Study the drawing (mm; zero at the part's minimum x, y, z) and answer. Round coordinates to 2 decimals unless told otherwise and drop trailing zeros. Write each loop counter-clockwise with the first axis right and the second up, starting at its lowest first coordinate (ties: lowest second). Pieces come first, ordered by that corner, then holes.
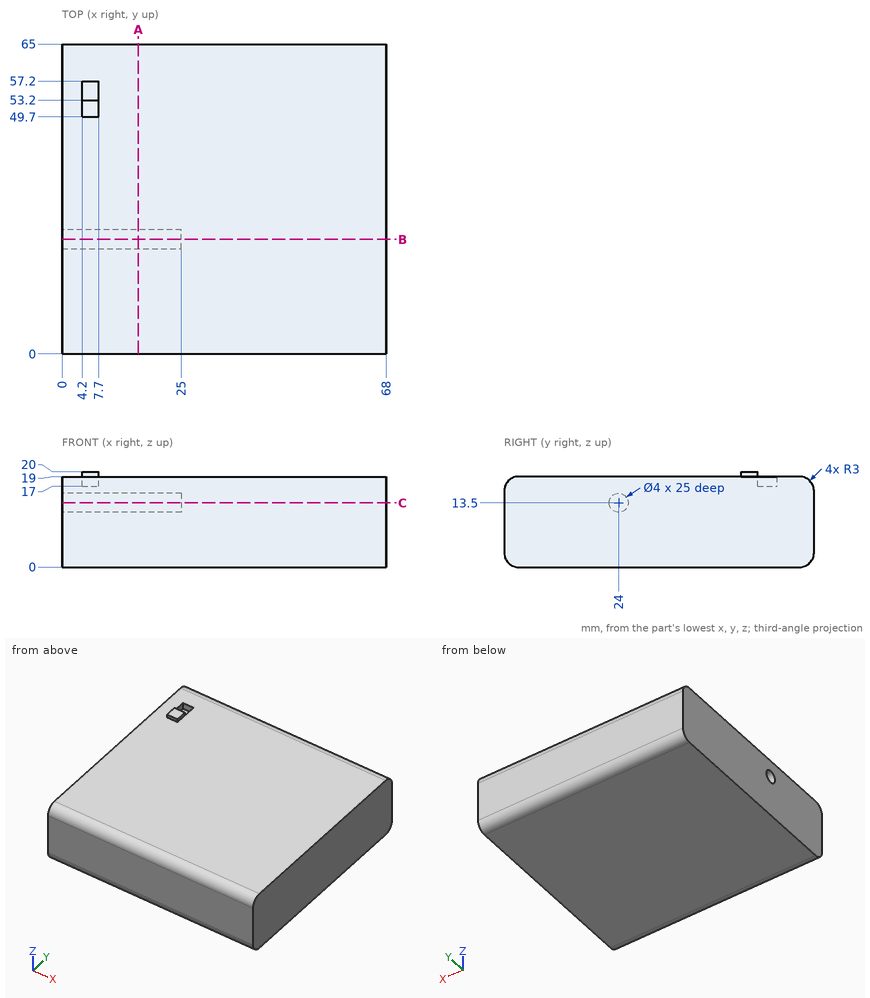
Q1. Find section C-C (z = 13.5). Determine the outline of the cut face in (x, y), plus the area to 3 significant figures.
Q2. Find section B-B (y = 24). Determine the outline of the cut face in (x, z).
Q3. Find the intervals of material crossed by L1, parallel to Z at x = 14, y = 24; L2, parallel to Z at x = 49, y = 6; L3, parallel to Y at x = 18.5, z = 13, in increasing order.
Q4. Find section A-A (x = 16). Determine the outline of the cut face in (y, z), plus the area to 3 significant figures.
Q5. Given pin 1 (3 mm diameter, centred on x = 5.5, y = 55.5, fed in from +Z); pin 2 (3 mm diameter, centred on y = 29.5, z = 14.5, fed in from -X); pin 3 (3.5 mm diameter, centred on x = 5.5, z = 18, fed in from +Y); pin 4 (1.2 mm diameter, centred on y = 24, z = 13, fed in from -X), each flat-ended and moving along its own axis, determine where each tip first touches the part or whether it passes through.
Report:
1. outline: (0, 0) - (68, 0) - (68, 65) - (0, 65) - (0, 26) - (25, 26) - (25, 22) - (0, 22) - close
1. area: 4,320 mm2
2. outline: (0, 0) - (68, 0) - (68, 19) - (0, 19) - (0, 15.5) - (25, 15.5) - (25, 11.5) - (0, 11.5) - close
3. L1: z = 0 to 11.5, 15.5 to 19
3. L2: z = 0 to 19
3. L3: y = 0 to 22.06, 25.94 to 65
4. outline: (0, 3) arc R3 ccw to (3, 0) - (62, 0) arc R3 ccw to (65, 3) - (65, 16) arc R3 ccw to (62, 19) - (3, 19) arc R3 ccw to (0, 16) - close; hole circle Ø4 at (24, 13.5)
4. area: 1,210 mm2
5. pin 1: stops at z = 19
5. pin 2: stops at x = 0
5. pin 3: stops at y = 64.99
5. pin 4: stops at x = 25
